Verification items for the finished model (mm, model axes). Round coordinates to 2 decimals unless told otherwise and drop trailing zeros. Write each loop counter-clockwise with the first axis right and the second up, starting at its lowest first coordinate (ties: lowest second). Pieces come first, ordered by that corner, then holes. Notation, with made-up numbers: M -31,53 L 16,53 A14 cw 16,64 Z; hole C 19.25,31 d2. An arc over 180 degrees is marked long. Answer in a Markdown table with one row per item. Add a question column.
1. Sectioned sample at C-C on y = 1.1. Record the cut outline in (x, z).
2. Sectioned sample at A-A on z = -21. Record the cut outline in (x, y), plus the area to 3 significant figures.
3. Material ranges on probe 1 along Z at (x, y) = (-21, 1.55); probe 2 along X at (y, z) = (0.9, -3.25); probe 3 along X at (y, z) = (0.1, -20), recorded low to high.
4. Sectioned sample at B-B on x = -2. Record the cut outline in (y, z), plus the area to 3 significant figures.
Autodesk Inventor part; units mm, degrees
ref_plane "YZ Plane" through (0, 0, 0) normal (1, 0, 0) x (0, 1, 0)
ref_plane "XZ Plane" through (0, 0, 0) normal (0, 1, 0) x (-1, 0, 0)
ref_plane "XY Plane" through (0, 0, 0) normal (0, 0, 1) x (1, 0, 0)
sketch "Sketch1" plane through (0, 0, 0) normal (0, 1, 0) x (-1, 0, 0)
  line L0 (0, 0) -> (23, 0)
  line L1 (23, 0) -> (23, -23)
  line L2 (23, -23) -> (0, -23)
  line L3 (0, -23) -> (0, 0)
  line L4 (23, 0) -> (21, 0)
  circle A0 centre (21, -2) radius 1.5
  circle A1 centre (2, -2) radius 1.5
  circle A2 centre (21, -21) radius 1.5
  circle A3 centre (2, -21) radius 1.5
  dimension "d0" = 23
  dimension "d1" = 23
  dimension "d4" = 3
extrude "Extrusion1" add sketch "Sketch1" along normal blind 2
properties part number "Mag_Sensor"
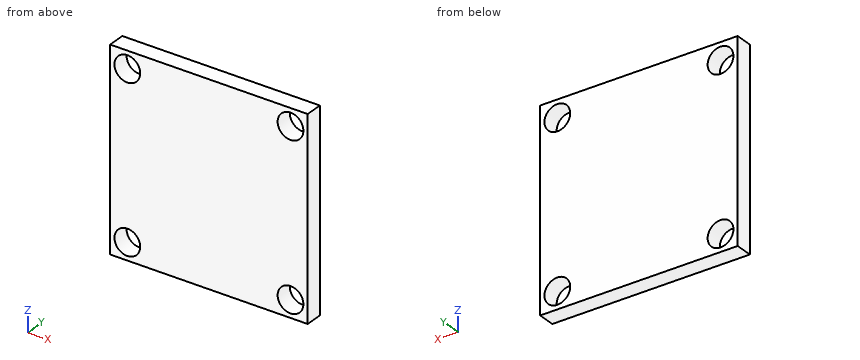
Geometry check:
| question | item | result |
|---|---|---|
| 1 | outline | M -23,-23 L 0,-23 L 0,0 L -23,0 Z; hole C -21,-21 d3; hole C -21,-2 d3; hole C -2,-21 d3; hole C -2,-2 d3 |
| 2 | outline | M -23,0 L -22.5,0 L -22.5,2 L -23,2 Z; M -19.5,0 L -3.5,0 L -3.5,2 L -19.5,2 Z; M -0.5,0 L 0,0 L 0,2 L -0.5,2 Z |
| 2 | area | 34.0 mm2 |
| 3 | probe 1 | z = -23 to -22.5, -19.5 to -3.5, -0.5 to 0 |
| 3 | probe 2 | x = -23 to -21.83, -20.17 to -2.83, -1.17 to 0 |
| 3 | probe 3 | x = -23 to -22.12, -19.88 to -3.12, -0.88 to 0 |
| 4 | outline | M 0,-23 L 2,-23 L 2,-22.5 L 0,-22.5 Z; M 0,-19.5 L 2,-19.5 L 2,-3.5 L 0,-3.5 Z; M 0,-0.5 L 2,-0.5 L 2,0 L 0,0 Z |
| 4 | area | 34.0 mm2 |
